The figure shows three views and two pictorial views of one solid part (mm, origin at its lowest corner). Answer the questions. A direction names the side the tool comes from. Coordinates: 2 decimals unless noted, no trailing zeros. Write each loop counter-clockwise with the first axis right and the second up, starting at its lowest first coordinate (ties: lowest second). Pieces come first, ordered by that corner, then holes.
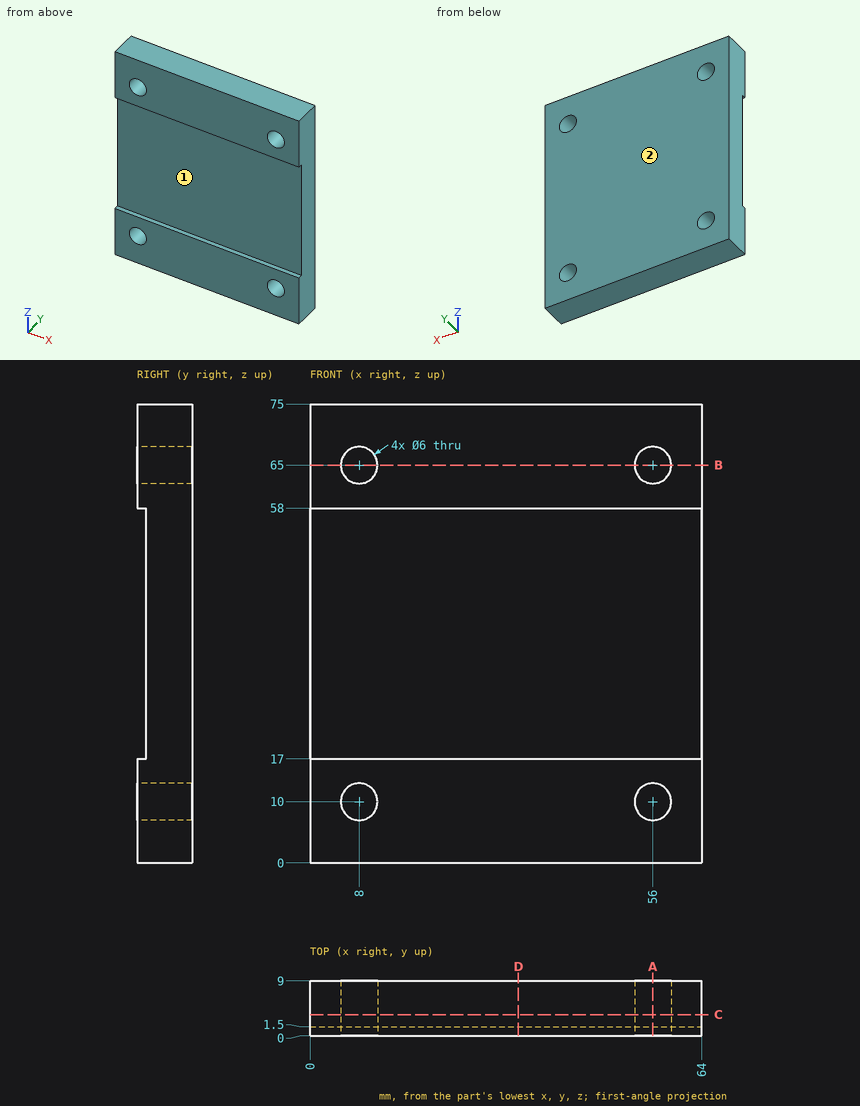
1. Find the intervals of material crossed by L1, parallel to Z at x = 56, y = 7.25; L2, parallel to X at y = 5.75, z = 11; L3, parallel to Z at x = 58, y = 3.5, in increasing order.
Results found:
L1: z = 0 to 7, 13 to 62, 68 to 75
L2: x = 0 to 5.17, 10.83 to 53.17, 58.83 to 64
L3: z = 0 to 7.76, 12.24 to 62.76, 67.24 to 75
2. Section B-B on z = 65 is taken. Give the vertices of the cut face in (x, y).
Results found:
outline: (0, 0) - (5, 0) - (5, 9) - (0, 9) - close; (11, 0) - (53, 0) - (53, 9) - (11, 9) - close; (59, 0) - (64, 0) - (64, 9) - (59, 9) - close
3. Section A-A on x = 56 is taken. Give the vertices of the cut face in (y, z), then the cut area to 4 significant figures.
Results found:
outline: (0, 0) - (9, 0) - (9, 7) - (0, 7) - close; (0, 13) - (9, 13) - (9, 62) - (0, 62) - (0, 58) - (1.5, 58) - (1.5, 17) - (0, 17) - close; (0, 68) - (9, 68) - (9, 75) - (0, 75) - close
area: 505.5 mm2
4. Flat-ended cylindrical pins translate along their axes: P1, Ø5, axis at x = 32, y = 2.5, coming from the -Z side; P2, Ø20.5, axis at x = 36, z = 28.5, coming from the -Y side. Find the tip coordinate at first contact, or state that the pin passes through.
Results found:
P1: stops at z = 0
P2: stops at y = 1.5
5. Section C-C on y = 3.5 is taken. Give the vertices of the cut face in (x, z), then the cut area to 3 significant figures.
Results found:
outline: (0, 0) - (64, 0) - (64, 75) - (0, 75) - close; hole circle Ø6 at (8, 10); hole circle Ø6 at (8, 65); hole circle Ø6 at (56, 10); hole circle Ø6 at (56, 65)
area: 4,690 mm2
6. A tool of negligible diameter and unlimited length cuts with its end or side. For the marked faces 1 and 2, from which of +Z, -Z, +X, -X, +Y, -Y can it reach the whole face along a straight path? Write none if from no direction.
Results found:
face 1: +X, -X, -Y
face 2: +Z, -Z, +X, -X, +Y
7. Section D-D on x = 34 is taken. Give the vertices of the cut face in (y, z).
Results found:
outline: (0, 0) - (9, 0) - (9, 75) - (0, 75) - (0, 58) - (1.5, 58) - (1.5, 17) - (0, 17) - close
